Geometry: final body of the model. Coordinates: model frame, mm. Give positions to 0.01 mm unless a question says otherwise; leave off trailing zeros. Write each loop counter-clockwise with the first axis right and the second up, starting at its lowest first coordinate (ties: lowest second). Pieces come first, ordered by that corner, then holes. Notation, with made-up numbers: (16.5, -32) -> (68.5, -32) arc R32 cw to (68.5, -3) -> close; hole circle Ø1 at (10.25, -22.75). An arc over 180 degrees is marked (long way). Use CSV: the item, a comma, the result in double quotes. Start each with the question number.
1) Section C-C (x = -214). Output: boundary loops of the cut face in (y, z).
2) Draft query along X for faces 1 (the face through (-86.67, -2.57, 12.23)), 2 (the face through (0, -6, 12)), 3 (the face through (-155, -12.7, 12)). Return one class per face: pulls with the +X half, pulls with the -X half, needs draft (parallel to the pull), parting line crosses it, or undercut.
3) Contact query for flat-ended pins moving along their axis: P1, Ø5, axis at y = 3.5, z = 20, coming from the -X side; P2, Ø2, axis at x = -224.5, z = 18.5, coming from the +Y side; P3, Ø1.9, axis at x = -2, z = 6.5, coming from the +Y side. Output: stop coordinate, or through.
4) Material intervals for line 1 (Y direction, x = -170.5, z = 8.5); line 2 (Y direction, x = -202.5, z = 14), sorted ascending. Write a range as [from, to].
5) Section B-B (y = 2.5). Count the separate pieces of the cut face and the enclosed holes in it, plus the area to 3 significant figures.
6) Section A-A (x = -6.35). Output: boundary loops of the cut face in (y, z), plus the area to 3 significant figures.
```python
from build123d import *

# Parameters (mm, degrees)
SKETCH1_W           = 304.8
SKETCH1_H           = 12.7
BOSS_EXTRUDE1_DEPTH = 24.13
SKETCH3_R           = 2.57175
CUT_EXTRUDE1_DEPTH  = 39.624
BOSS_EXTRUDE2_DEPTH = 24.13


with BuildPart() as part:
    # Sketch1 → Boss-Extrude1 (new body)
    with BuildSketch(Plane.XY):
        with Locations((-152.4, -6.35)):
            Rectangle(SKETCH1_W, SKETCH1_H)
    extrude(amount=BOSS_EXTRUDE1_DEPTH)

    # Sketch3 → Cut-Extrude1 (cut)
    with BuildSketch(Plane.XY.offset(24.13)):
        with Locations((-26.416, 0)):
            Circle(SKETCH3_R)
        with Locations((-46.482, 0)):
            Circle(SKETCH3_R)
        with Locations((-66.548, 0)):
            Circle(SKETCH3_R)
        with Locations((-86.614, 0)):
            Circle(SKETCH3_R)
        with Locations((-106.68, 0)):
            Circle(SKETCH3_R)
        with Locations((-126.746, 0)):
            Circle(SKETCH3_R)
        with Locations((-146.812, 0)):
            Circle(SKETCH3_R)
        with Locations((-166.878, 0)):
            Circle(SKETCH3_R)
        with Locations((-186.944, 0)):
            Circle(SKETCH3_R)
        with Locations((-6.35, 0)):
            Circle(SKETCH3_R)
        with Locations((-207.01, 0)):
            Circle(SKETCH3_R)
        with Locations((-227.076, 0)):
            Circle(SKETCH3_R)
        with Locations((-247.142, 0)):
            Circle(SKETCH3_R)
        with Locations((-267.208, 0)):
            Circle(SKETCH3_R)
        with Locations((-287.274, 0)):
            Circle(SKETCH3_R)
    extrude(amount=-CUT_EXTRUDE1_DEPTH, mode=Mode.SUBTRACT)

    # Sketch4 → Boss-Extrude2 (add)
    with BuildSketch(Plane(origin=(0, 0, 0), x_dir=(-1, 0, 0), z_dir=(0, 0, -1))):
        Polygon((16.383, 6.35), (8.92175, 0), (23.84425, 0), align=None)
        Polygon((36.449, 6.35), (28.98775, 0), (43.91025, 0), align=None)
        Polygon((63.97625, 0), (56.515, 6.35), (49.05375, 0), align=None)
        Polygon((84.04225, 0), (76.581, 6.35), (69.11975, 0), align=None)
        Polygon((104.10825, 0), (96.647, 6.35), (89.18575, 0), align=None)
        Polygon((124.17425, 0), (116.713, 6.35), (109.25175, 0), align=None)
        Polygon((144.24025, 0), (136.779, 6.35), (129.31775, 0), align=None)
        Polygon((164.30625, 0), (156.845, 6.35), (149.38375, 0), align=None)
        Polygon((184.37225, 0), (176.911, 6.35), (169.44975, 0), align=None)
        Polygon((204.43825, 0), (196.977, 6.35), (189.51575, 0), align=None)
        Polygon((224.50425, 0), (217.043, 6.35), (209.58175, 0), align=None)
        Polygon((244.57025, 0), (237.109, 6.35), (229.64775, 0), align=None)
        Polygon((264.63625, 0), (257.175, 6.35), (249.71375, 0), align=None)
        Polygon((284.70225, 0), (277.241, 6.35), (269.77975, 0), align=None)
        Polygon((304.76825, 0), (297.307, 6.35), (289.84575, 0), align=None)
    extrude(amount=-BOSS_EXTRUDE2_DEPTH)


solid = part.part
```
Answers follow:
1,outline,"(-12.7, 0) -> (3.76, 0) -> (3.76, 24.13) -> (-12.7, 24.13) -> close"
2,face 1,"undercut"
2,face 2,"pulls with the +X half"
2,face 3,"needs draft"
3,P1,"stops at x = -303.59"
3,P2,"stops at y = 0.85"
3,P3,"stops at y = 0"
4,line 1,"y = [-12.7, 0.89]"
4,line 2,"y = [-12.7, 1.65]"
5,separate pieces,"15"
5,enclosed holes,"0"
5,area,"3,270 mm^2"
6,outline,"(-12.7, 0) -> (-2.57, 0) -> (-2.57, 24.13) -> (-12.7, 24.13) -> close"
6,area,"244 mm^2"
